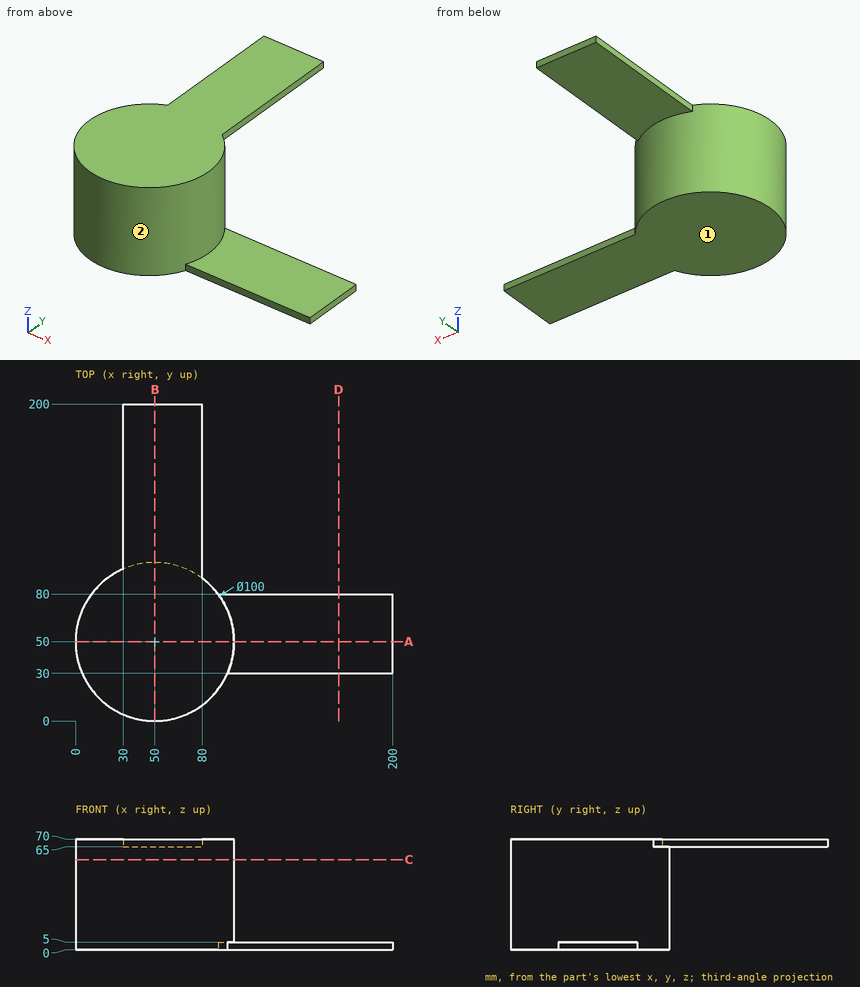
Study the drawing (mm; zero at the part's minimum x, y, z) and answer. A direction names the side the tool comes from. Round coordinates to 2 decimals unless told otherwise and drop trailing zeros. Write each loop counter-clockwise with the first axis right and the second up, starting at its lowest first coordinate (ties: lowest second). Pieces come first, ordered by that corner, then holes.
Q1. Straight lines are drawn through the part: line 1 (X direction, y = 50, z = 17); line 2 (Z direction, x = 70.5, y = 139); line 3 (Y direction, x = 83, z = 50.5). For each, find the intervals that lie inside material, in ascending order.
Values:
line 1: x = 0 to 100
line 2: z = 65 to 70
line 3: y = 12.44 to 87.56
Q2. Find section C-C on z = 57. Determine the outline of the cut face in (x, y).
Values:
outline: circle Ø100 at (50, 50)
Q3. Find section B-B on x = 50. Determine the outline of the cut face in (y, z), and give its area (3 significant figures).
Values:
outline: (0, 0) - (100, 0) - (100, 65) - (200, 65) - (200, 70) - (0, 70) - close
area: 7,500 mm2
Q4. A tool of negligible diameter and unlimited length cuts with its end or side. For the marked faces 1 and 2, from which of +Z, -Z, +X, -X, +Y, -Y can it reach the whole face along a straight path? Write none if from no direction.
Values:
face 1: -Z, +X, -X, +Y, -Y
face 2: none
Q5. Find section D-D on x = 166. Determine the outline of the cut face in (y, z).
Values:
outline: (30, 0) - (80, 0) - (80, 5) - (30, 5) - close
Q6. Flat-ended cylindrical pins translate along their axes: P1, Ø6, axis at y = 87.5, z = 43, coming from the +X side; P2, Ø1.5, axis at y = 153.5, z = 68, coming from the -X side; P3, Ø1.5, axis at x = 157, z = 1.5, coming from the -Y side. Find the tip coordinate at first contact, or state that the pin passes through.
Values:
P1: stops at x = 86.19
P2: stops at x = 30
P3: stops at y = 30
Q7. Find section A-A on y = 50. Determine the outline of the cut face in (x, z), and give its area (3 significant figures).
Values:
outline: (0, 0) - (200, 0) - (200, 5) - (100, 5) - (100, 70) - (0, 70) - close
area: 7,500 mm2
